Source: three-view drawing plus pictorial views. Frame: mm from the lowest corner of the part. A direction names the side the tool comes from. Round coordinates to 2 decimals unless told otherwise and drop trailing zeros. Order: outer loops, then holes, each group sorted by start corner. A loop starts at its lowest first (then second) coordinate and runs counter-clockwise, first axis right, second up. Notation, with made-up numbers: (83, 73) - (117, 73) arc R5 cw to (117, 77) - close; hole circle Ø7 at (36.5, -0.75). An arc over 180 degrees is marked (long way). One line per item, written item: value. Start each with the question number.
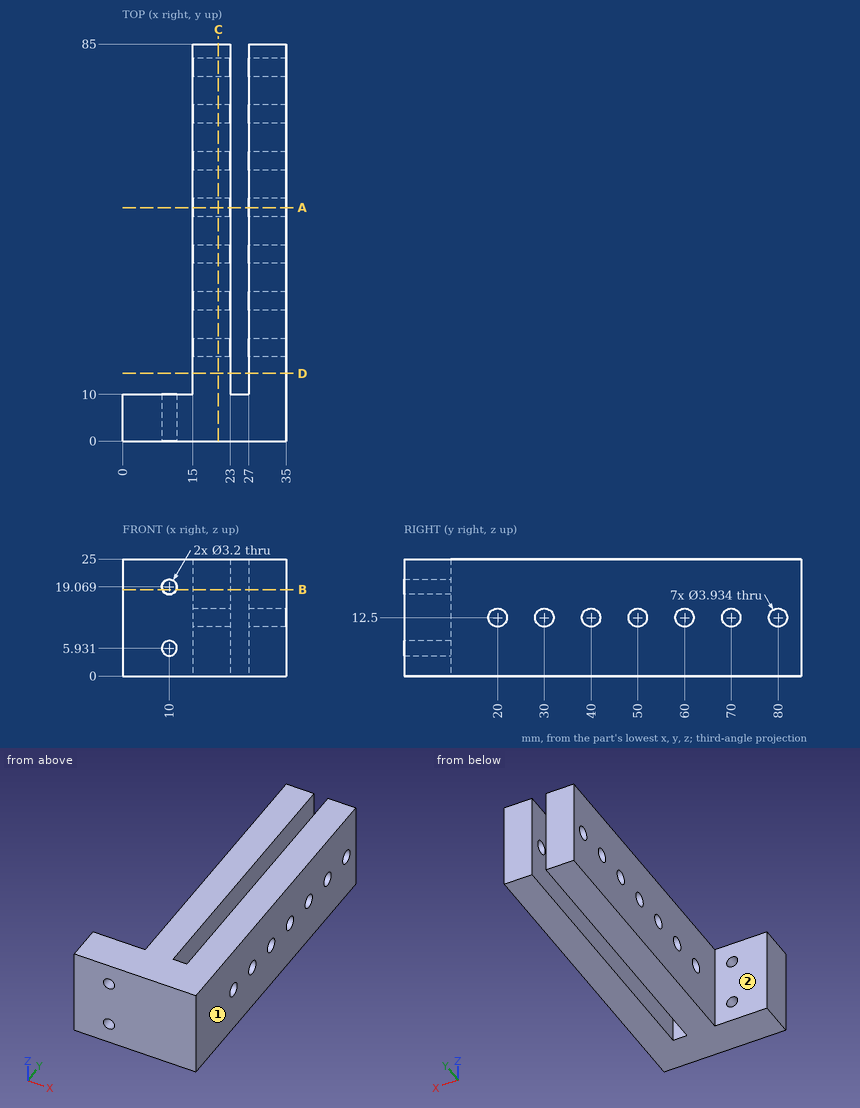
Item 1: Reachability of the marked faces 1 and 2 from +Z, -Z, +X, -X, +Y, -Y: full face, straight path, thin tool, end or side. Return the list, or none.
Item 2: Section query D-D on y = 14.5. Return loops of the section in (x, z), and give its area (3 significant figures).
Item 3: Section query A-A on y = 50. Return loops of the section in (x, z), and give its area (3 significant figures).
Item 4: First-contact query: pin 1 Ø3 at (y, z) = (70, 12.5) entering from +X; pin 2 Ø2 at (x, z) = (25, 7) entering from +Y; pin 3 Ø6.5 at (y, z) = (40, 12.5) entering from -X. Flat tips, straight axial feed; report the tip coordinate or a pass-through.
Item 5: Section query C-C on x = 20.5. Return loops of the section in (y, z), and give its area (3 significant figures).
Item 6: Section query B-B on z = 18.5. Return loops of the section in (x, y) (1 decimal), and give its area (3 significant figures).
Item 7: Line query: L1, parallel to X at y = 76, z = 21.5; L2, parallel to Y at x = 9, z = 10.75; L3, parallel to Z at x = 28.5, y = 29 (1 decimal). Output: solid intervals per line, ascending.
Geometry results:
1. face 1: +Z, -Z, +X, +Y, -Y
1. face 2: +Z, -Z, -X, +Y
2. outline: (15, 0) - (23, 0) - (23, 25) - (15, 25) - close; (27, 0) - (35, 0) - (35, 25) - (27, 25) - close
2. area: 400 mm^2
3. outline: (15, 0) - (23, 0) - (23, 10.53) - (15, 10.53) - close; (15, 14.47) - (23, 14.47) - (23, 25) - (15, 25) - close; (27, 0) - (35, 0) - (35, 10.53) - (27, 10.53) - close; (27, 14.47) - (35, 14.47) - (35, 25) - (27, 25) - close
3. area: 337 mm^2
4. pin 1: passes through
4. pin 2: stops at y = 10
4. pin 3: stops at x = 15
5. outline: (0, 0) - (85, 0) - (85, 25) - (0, 25) - close; hole circle Ø3.93 at (20, 12.5); hole circle Ø3.93 at (30, 12.5); hole circle Ø3.93 at (40, 12.5); hole circle Ø3.93 at (50, 12.5); hole circle Ø3.93 at (60, 12.5); hole circle Ø3.93 at (70, 12.5); hole circle Ø3.93 at (80, 12.5)
5. area: 2,040 mm^2
6. outline: (0, 0) - (8.5, 0) - (8.5, 10) - (0, 10) - close; (11.5, 0) - (35, 0) - (35, 85) - (27, 85) - (27, 10) - (23, 10) - (23, 85) - (15, 85) - (15, 10) - (11.5, 10) - close
6. area: 1,520 mm^2
7. L1: x = 15 to 23, 27 to 35
7. L2: y = 0 to 10
7. L3: z = 0 to 10.8, 14.2 to 25
